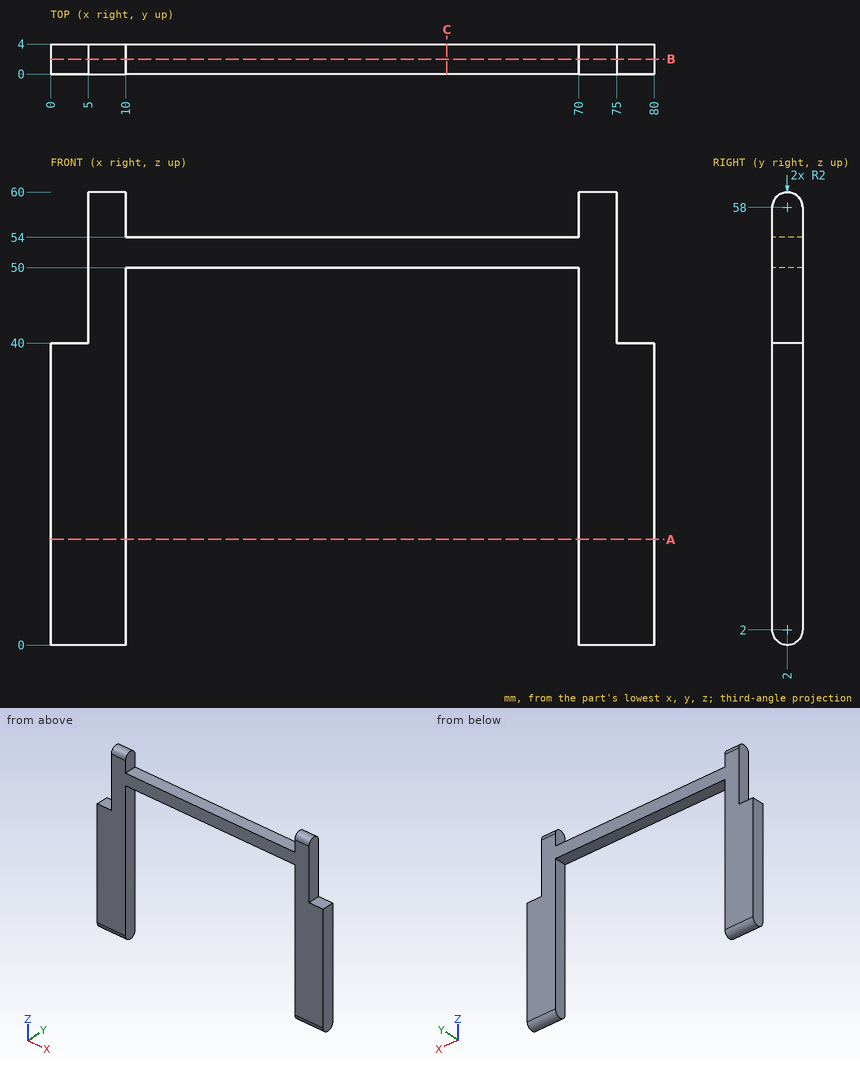
Answer from the drawing. Dimensions are ordinates in mm from the lowest x, y and z of the part. Give positions to 0.01 mm unless a question says otherwise; leave off trailing zeros. Loops run counter-clockwise (first coordinate to the right, second up) from the corner with the lowest first, then second, coordinate; pieces in that order, holes last. Notation, with made-up numbers: (-5, 40) -> (20, 40) arc R25 cw to (20, 72) -> close; hole circle Ø3 at (89.25, 52.5). An arc over 180 degrees is marked (long way). One line per question, with ' | ' between items. Start each with the question number.
1) Each of these flat-tipped pins is pushed along its axis until it touches: pin 1 (1 mm diameter, centred on x = 60.5, y = 2, fed in from -Z); pin 2 (1.2 mm diameter, centred on x = 2.5, y = 3, fed in from +Z); pin 3 (1.2 mm diameter, centred on y = 1.5, z = 52, fed in from +X). Where does it stop, or does it pass through?
2) Straight lines are drawn through the part: L1, parallel to X at y = 2.55, z = 13.5; L2, parallel to X at y = 1.2, z = 47.5; L3, parallel to Z at x = 15, y = 3.45. For each, find the intervals that lie inside material, in ascending order.
3) Section C-C, the plane x = 52.5 is taken. Determine the outline of the cut face in (y, z), then the cut area to 3 significant figures.
4) Section A-A, the plane z = 14 is taken. Determine the outline of the cut face in (x, y).
5) Section B-B, the plane y = 2 is taken. Determine the outline of the cut face in (x, z), then the cut area to 3 significant figures.
Resolved:
1) pin 1: z = 50 | pin 2: z = 40 | pin 3: x = 75
2) L1: 0 to 10, 70 to 80 | L2: 5 to 10, 70 to 75 | L3: 50 to 54
3) outline: (0, 50) -> (4, 50) -> (4, 54) -> (0, 54) -> close | area: 16.0 mm2
4) outline: (0, 0) -> (10, 0) -> (10, 4) -> (0, 4) -> close; (70, 0) -> (80, 0) -> (80, 4) -> (70, 4) -> close
5) outline: (0, 0) -> (10, 0) -> (10, 50) -> (70, 50) -> (70, 0) -> (80, 0) -> (80, 40) -> (75, 40) -> (75, 60) -> (70, 60) -> (70, 54) -> (10, 54) -> (10, 60) -> (5, 60) -> (5, 40) -> (0, 40) -> close | area: 1,240 mm2
